Autodesk Inventor part; units mm, degrees
ref_plane "YZ Plane" through (0, 0, 0) normal (1, 0, 0) x (0, 1, 0)
ref_plane "XZ Plane" through (0, 0, 0) normal (0, 1, 0) x (-1, 0, 0)
ref_plane "XY Plane" through (0, 0, 0) normal (0, 0, 1) x (1, 0, 0)
sketch "Sketch1" plane through (0, 0, 0) normal (0, 1, 0) x (-1, 0, 0)
  line L0 (5, 37.5) -> (-5, 37.5)
  line L1 (-5, 37.5) -> (-5, -37.5)
  line L2 (-5, -37.5) -> (5, -37.5)
  line L3 (5, -37.5) -> (5, 37.5)
  point P0 (0, 0)
  point P1 (5, 0)
  point P2 (0, 37.5)
  dimension "d0" = 10
  dimension "d1" = 75
extrude "Extrusion1" add sketch "Sketch1" along normal blind 12
sketch "Sketch2" plane through (5, 0, 37.5) normal (1, 0, 0) x (0, 0, -1)
  line L0 (7, 0) -> (68, 0)
  line L1 (68, 0) -> (68, 7.5)
  line L2 (67, 8.5) -> (8, 8.5)
  line L3 (7, 7.5) -> (7, 0)
  line L4 (0, 0) -> (75, 0)
  arc A0 (8, 8.5) -> (7, 7.5) centre (8, 7.5) ccw
  arc A1 (68, 7.5) -> (67, 8.5) centre (67, 7.5) ccw
  point P0 (37.5, 0)
  point P1 (37.5, 0)
  dimension "d4" = 61
  dimension "d5" = 8.5
  dimension "d6" = 1
extrude "Extrusion2" cut sketch "Sketch2" against normal through all
sketch "Sketch3" plane through (0, 12, 0) normal (0, 1, 0) x (1, 0, 0)
  line L0 (-5, 37.5) -> (-5, -37.5)
  point P0 (0, 0)
  point P1 (-1, 33.5)
  point P2 (-1, -33.5)
  dimension "d9" = 67
  dimension "d19" = 4
  dimension "d20" = 33.5
hole "Hole1" at (-1, 12, -33.5) at (-1, 12, 33.5) direction (0, -1, 0) diameter 3.2 end through all
fillet "Fillet1" radius 4 2 edges at (-5, 6, 37.5) (-5, 6, -37.5)
properties part number "phone_clamp"
Input: part model. Units: mm. Frame: model coordinates. A direction names the side the tool comes from. Coordinates: 2 decimals unless noted, no trailing zeros. Write each loop counter-clockwise with the first axis right and the second up, starting at its lowest first coordinate (ties: lowest second). Pieces come first, ordered by that corner, then holes. Notation, with made-up numbers: (-2, 49.5) -> (34, 49.5) arc R34 cw to (34, 81.5) -> close; hole circle Ø5 at (-10.75, 52). An arc over 180 degrees is marked (long way). Write each question's results on one line, items separated by ' | '.
Item 1: Section query B-B on y = 1.5. Return loops of the section in (x, z), plus the area to 3 significant figures.
Conclusion:
outline: (-5, -33.5) arc R4 ccw to (-1, -37.5) -> (5, -37.5) -> (5, -30.5) -> (-5, -30.5) -> close; (-5, 30.5) -> (5, 30.5) -> (5, 37.5) -> (-1, 37.5) arc R4 ccw to (-5, 33.5) -> close; hole circle Ø3.2 at (-1, -33.5); hole circle Ø3.2 at (-1, 33.5) | area: 117 mm^2
Item 2: Section query A-A on y = 9.5. Return loops of the section in (x, z).
Conclusion:
outline: (-5, -33.5) arc R4 ccw to (-1, -37.5) -> (5, -37.5) -> (5, 37.5) -> (-1, 37.5) arc R4 ccw to (-5, 33.5) -> close; hole circle Ø3.2 at (-1, -33.5); hole circle Ø3.2 at (-1, 33.5)
Item 3: Section query D-D on z = -20. Return loops of the section in (x, y), plus the area to 3 significant figures.
Conclusion:
outline: (-5, 8.5) -> (5, 8.5) -> (5, 12) -> (-5, 12) -> close | area: 35.0 mm^2
Item 4: Pin query (flat end, axial travel): pin 1 Ø2 at (y, z) = (7, 2) entering from +X. Return the tip coordinate at first contact, or that it passes through.
Conclusion:
pin 1: passes through
Item 5: Set-up query: faces 1 (the flat face through (1, 0, -34)), 2 (the flat face through (0, 4, -30.5)). Return all of +Z, -Z, +X, -X, +Y, -Y with unobstructed straight access to the full face (end or side cutting, diameter ignored); none if empty.
Conclusion:
face 1: +Z, -Z, +X, -X, -Y | face 2: +X, -X, -Y
Item 6: Mould query, pull axis X, two halves, no side actions, for faces 3 (the flat face through (-5, 9, 0)), 4 (the cylindrical face through (-1.07, 5.92, -35.1)), 5 (the cylindrical face through (-1.07, 5.92, 31.9)), 6 (the flat face through (0, 8.5, 0)). Classes: +X half, -X half, draft (parallel to the pull), parting line (faces both ways), or undercut.
Conclusion:
face 3: -X half | face 4: undercut | face 5: undercut | face 6: draft
Item 7: Material intervals for probe 1 along Z at (x, y) = (-1, 6.5); probe 2 along Z at (x, y) = (-1, 9.25); probe 3 along X at (y, z) = (9, -33.5), sorted ascending.
Conclusion:
probe 1: z = -37.5 to -35.1, -31.9 to -30.5, 30.5 to 31.9, 35.1 to 37.5 | probe 2: z = -37.5 to -35.1, -31.9 to 31.9, 35.1 to 37.5 | probe 3: x = -5 to -2.6, 0.6 to 5
Item 8: Section query C-C on x = 3. Return loops of the section in (y, z), plus the area to 3 significant figures.
Conclusion:
outline: (0, -37.5) -> (12, -37.5) -> (12, 37.5) -> (0, 37.5) -> (0, 30.5) -> (7.5, 30.5) arc R1 cw to (8.5, 29.5) -> (8.5, -29.5) arc R1 cw to (7.5, -30.5) -> (0, -30.5) -> close | area: 382 mm^2
